Verification items for the finished model (mm, model axes). Face numbers are marked on the shaded views. A direction names the side the tool comes from. Round coordinates to 2 decimals unless told otherwise and drop trailing zeros. Write each loop counter-clockwise with the first axis right and the second up, starting at its lowest first coordinate (ties: lowest second). Pieces come first, ordered by that corner, then holes. Notation, with made-up numbers: M 18.25,-22 L 49.25,-22 A22 cw 49.25,16 Z; hole C 30,8.25 d6. An arc over 180 degrees is marked long. Use a Markdown table: item, result. Add a question column.
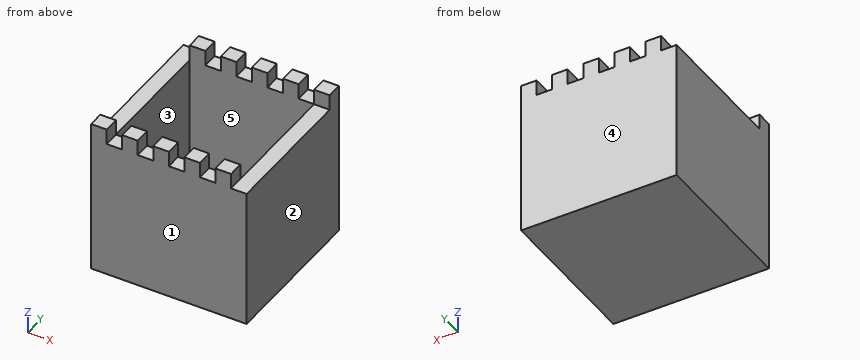
from build123d import *

# Parameters (mm, degrees)
F0_W     = 25.4
F0_H     = 25.4
F1_DEPTH = 25.4
F3_DEPTH = 2.54
F4_W     = 20.32
F4_H     = 20.32
F5_DEPTH = 20.32


with BuildPart() as f1:
    # F0 (on Top) → F1 (new body)
    with BuildSketch(Plane.XY):
        Rectangle(F0_W, F0_H)
    extrude(amount=F1_DEPTH)

    # F2 (on face) → F3 (cut)
    with BuildSketch(Plane.XY.offset(25.4)):
        Polygon((12.7, -10.16), (12.7, 10.16), (10.16, 10.16), (10.16, 12.7), (7.62, 12.7), (7.62, 10.16), (5.08, 10.16), (5.08, 12.7), (2.54, 12.7), (2.54, 10.16), (0, 10.16), (0, 12.7), (-2.54, 12.7), (-2.54, 10.16), (-5.08, 10.16), (-5.08, 12.7), (-7.62, 12.7), (-7.62, 10.16), (-10.16, 10.16), (-10.16, 12.7), (-12.7, 12.7), (-12.7, 10.16), (-12.7, -10.16), (-10.16, -10.16), (-10.16, -12.7), (-7.62, -12.7), (-7.62, -10.16), (-5.08, -10.16), (-5.08, -12.7), (-2.54, -12.7), (-2.54, -10.16), (0, -10.16), (0, -12.7), (2.54, -12.7), (2.54, -10.16), (5.08, -10.16), (5.08, -12.7), (7.62, -12.7), (7.62, -10.16), (10.16, -10.16), (10.16, -12.7), (12.7, -12.7), align=None)
    extrude(amount=-F3_DEPTH, mode=Mode.SUBTRACT)

    # F4 (on face) → F5 (cut)
    with BuildSketch(Plane.XY.offset(22.86)):
        Rectangle(F4_W, F4_H)
    extrude(amount=-F5_DEPTH, mode=Mode.SUBTRACT)


solid = f1.part
1. Release check for a two-part mould opening along Y. For the marked faces 1, 2 and 3 record: +Y half, -Y half, draft (parallel to the pull), parting line (faces both ways), or undercut.
2. Scan lines: line 1 along X through (y, z) = (4.5, 16.5); line 2 along Z through (x, y) = (-0.75, -7.75). Record each from-to range of solid material in increasing order. Write a range as from..to.
3. Cross-section at C-C on y = 0.75. Enter the section's corners in (x, z).
4. Access from +Z, -Z, +X, -X, +Y, -Y to the whole of each face (thin tool, end or side, straight path). Record for the marked faces 4 and 5.
5. Depth check by flat-ended pin: pin 1 Ø2 at (y, z) = (-12, 24.5) entering from +X; pin 2 Ø5 at (x, y) = (0, -6) entering from +Z; pin 3 Ø2 at (x, y) = (9, 12) entering from +Z. Enter the tip coordinate at first touch or a pass-through.
6. Cross-section at B-B on z = 21.25. Enter the section's corners in (x, y), plus the area to 3 significant figures.
7. Cross-section at A-A on x = 0.75. Enter the section's corners in (y, z).
8. Cross-section at D-D on x = -11. Enter the section's corners in (y, z), plus the area to 3 significant figures.
Answer:
| question | item | result |
|---|---|---|
| 1 | face 1 | -Y half |
| 1 | face 2 | draft |
| 1 | face 3 | undercut |
| 2 | line 1 | x = -12.7..-10.16, 10.16..12.7 |
| 2 | line 2 | z = 0..2.54 |
| 3 | outline | M -12.7,0 L 12.7,0 L 12.7,22.86 L 10.16,22.86 L 10.16,2.54 L -10.16,2.54 L -10.16,22.86 L -12.7,22.86 Z |
| 4 | face 4 | +Z, -Z, +X, -X, +Y |
| 4 | face 5 | +Z |
| 5 | pin 1 | stops at x = 10.16 |
| 5 | pin 2 | stops at z = 2.54 |
| 5 | pin 3 | stops at z = 22.86 |
| 6 | outline | M -12.7,-12.7 L 12.7,-12.7 L 12.7,12.7 L -12.7,12.7 Z; hole M -10.16,-10.16 L 10.16,-10.16 L 10.16,10.16 L -10.16,10.16 Z |
| 6 | area | 232 mm^2 |
| 7 | outline | M -12.7,0 L 12.7,0 L 12.7,25.4 L 10.16,25.4 L 10.16,2.54 L -10.16,2.54 L -10.16,22.86 L -12.7,22.86 Z |
| 8 | outline | M -12.7,0 L 12.7,0 L 12.7,22.86 L -10.16,22.86 L -10.16,25.4 L -12.7,25.4 Z |
| 8 | area | 587 mm^2 |
